Can you work these out from the drawing? Everything is in mm from the part's minimum corner. A direction names the side the tool comes from. Coordinates: 2 decimals unless noted, no trailing zeros. Order: outer loops, then holes, each group sorted by start corner. A loop starts at its lowest first (then second) coordinate and runs counter-clockwise, first axis right, second up. Notation, with made-up numbers: (-29.5, -20) -> (-9.5, -20) arc R30 ccw to (-9.5, 18) -> close; hole circle Ø11 at (4.25, -16.75). An arc over 180 degrees is marked (long way). Put each result on its own line as item: value. Start each with the question number.
Q1. We'd pull the mould along Y, two halves only. Please class the marked faces 5, 6 and 7: +Y half, -Y half, draft (parallel to the pull), parting line (faces both ways), or undercut.
Q2. If we section it at D-D (z = 3.75): Please give me the cut outline in (x, y), and give its area (3 significant figures).
Q3. If we section it at C-C (x = 1.25): Please give me the cut outline in (y, z) (3 decimals).
Q4. If we section it at A-A (y = 8): Please give me the cut outline in (x, z) (3 decimals), and give its area (3 significant figures).
Q5. Will these pins go through, and if not, where does the flat tip stop? pin 1 (5 mm diameter, centred on y = 5, z = 13, fed in from -X); pin 2 (2 mm diameter, centred on x = 3, z = 8, fed in from -Y) (3 decimals); pin 3 (2 mm diameter, centred on x = 2.5, z = 9.5, fed in from +Y) (3 decimals); pin 4 (1.5 mm diameter, centred on x = 1, y = 9.5, fed in from +Z).
Q6. For the marked faces 1, 2, 3 and 4, which set-ups out of +Z, -Z, +X, -X, +Y, -Y let a thin tool reach every point of the face, with its end or its side?
Q7. If we section it at B-B (z = 8): Please give me the cut outline in (x, y) (3 decimals).
Q8. Please list where these lines run through material, in increasing order: line 1 along Z through (x, y) = (4.25, 8) (3 decimals); line 2 along Z through (x, y) = (4.5, 8) (3 decimals); line 3 along Y through (x, z) = (2.5, 8) (3 decimals).
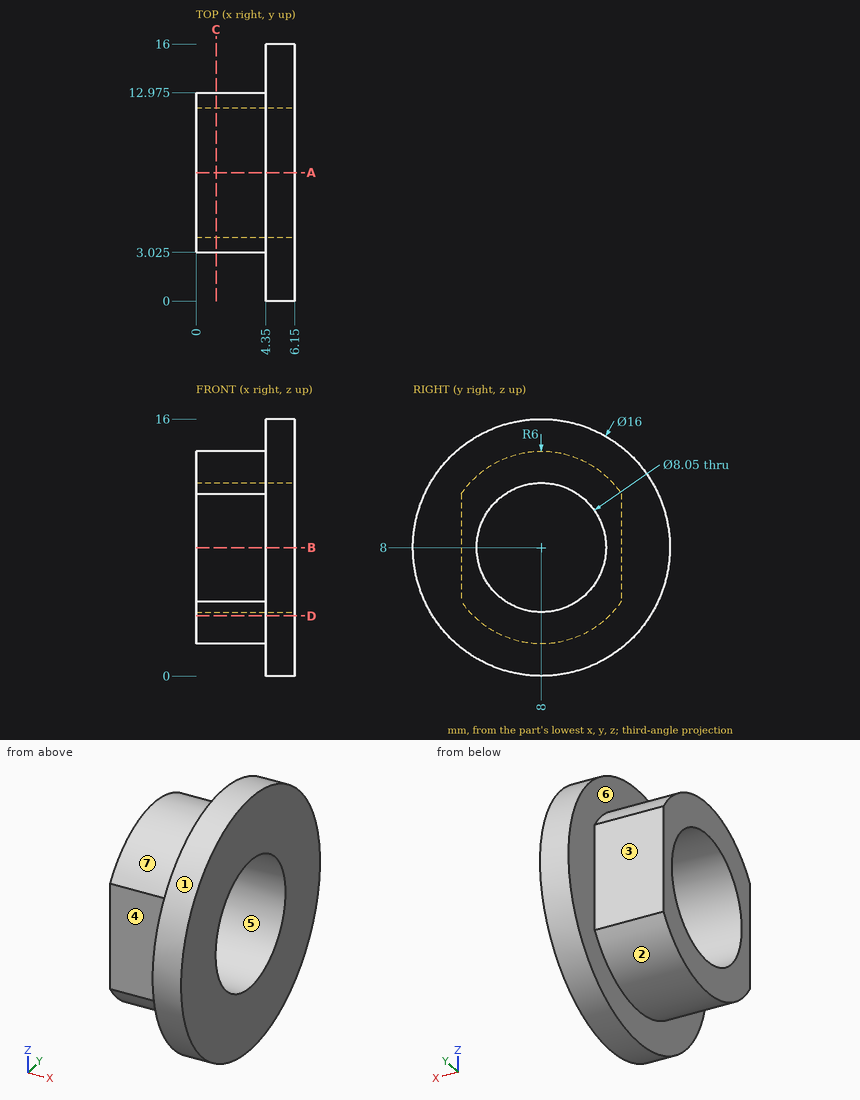
The answers:
1. face 5: undercut
1. face 6: draft
1. face 7: parting line
2. outline: (0, 3.76) -> (4.35, 3.76) -> (4.35, 1.22) -> (6.15, 1.22) -> (6.15, 14.78) -> (4.35, 14.78) -> (4.35, 12.24) -> (0, 12.24) -> close
2. area: 61.2 mm^2
3. outline: (3.025, 4.646) arc R6 ccw to (12.975, 4.646) -> (12.975, 11.354) arc R6 ccw to (3.025, 11.354) -> close; hole circle Ø8.05 at (8, 8)
4. outline: (0, 2) -> (4.35, 2) -> (4.35, 0) -> (6.15, 0) -> (6.15, 3.975) -> (0, 3.975) -> close; (0, 12.025) -> (6.15, 12.025) -> (6.15, 16) -> (4.35, 16) -> (4.35, 14) -> (0, 14) -> close
4. area: 31.5 mm^2
5. pin 1: x = 0
5. pin 2: y = 3.025
5. pin 3: y = 12.975
5. pin 4: z = 13.95
6. face 1: +X, -X
6. face 2: -Z, -X
6. face 3: +Z, -Z, -X, +Y
6. face 4: +Z, -Z, -X, -Y
7. outline: (0, 3.025) -> (4.35, 3.025) -> (4.35, 0) -> (6.15, 0) -> (6.15, 3.975) -> (0, 3.975) -> close; (0, 12.025) -> (6.15, 12.025) -> (6.15, 16) -> (4.35, 16) -> (4.35, 12.975) -> (0, 12.975) -> close
8. line 1: 2 to 3.975, 12.025 to 14
8. line 2: 0 to 3.975, 12.025 to 16
8. line 3: 3.025 to 3.975, 12.025 to 12.975
